For this review, take the finished solid that the model builds, in its own axes (mm). A direction names the side the tool comes from. Give positions to 0.01 mm unless a question says otherwise; leave off trailing zeros. Order: outer loops, then holes, each group sorted by start corner. A loop starts at its lowest first (then second) coordinate and runs counter-clockwise, first axis right, second up. Notation, with made-up numbers: (31, 71.25) - (47, 71.25) arc R26 cw to (47, 101.25) - close; hole circle Ø1 at (-18.75, -28). An arc over 180 degrees is marked (long way). Answer as a JSON object with one key per item and string values. Group by question number.
from build123d import *

# Parameters (mm, degrees)
F0_R     = 1.5
F0_R_2   = 4.5
F1_DEPTH = 2


with BuildPart() as f1:
    # F0 (on Top) → F1 (new body)
    with BuildSketch(Plane.XY):
        with BuildLine():
            ThreePointArc((-8.332531, 2.986763), (-11.332531, -0.013237), (-8.332531, -3.013237))
            Line((-8.332531, -3.013237), (-7.332531, -3.013237))
            ThreePointArc((-7.332531, -3.013237), (-4.504103, -4.184809), (-3.332531, -7.013237))
            Line((-3.332531, -7.013237), (-3.332531, -8.013237))
            ThreePointArc((-3.332531, -8.013237), (-0.332531, -11.013237), (2.667469, -8.013237))
            Line((2.667469, -8.013237), (2.667469, -7.013237))
            ThreePointArc((2.667469, -7.013237), (3.839042, -4.184809), (6.667469, -3.013237))
            Line((6.667469, -3.013237), (7.667469, -3.013237))
            ThreePointArc((7.667469, -3.013237), (10.667469, -0.013237), (7.667469, 2.986763))
            Line((7.667469, 2.986763), (6.667469, 2.986763))
            ThreePointArc((6.667469, 2.986763), (3.839042, 4.158336), (2.667469, 6.986763))
            Line((2.667469, 6.986763), (2.667469, 7.986763))
            ThreePointArc((2.667469, 7.986763), (-0.332531, 10.986763), (-3.332531, 7.986763))
            Line((-3.332531, 7.986763), (-3.332531, 6.986763))
            ThreePointArc((-3.332531, 6.986763), (-4.504103, 4.158336), (-7.332531, 2.986763))
            Line((-7.332531, 2.986763), (-8.332531, 2.986763))
        make_face()
        with Locations((-0.332531, -8.013237)):
            Circle(F0_R, mode=Mode.SUBTRACT)
        with Locations((-8.332531, -0.013237)):
            Circle(F0_R, mode=Mode.SUBTRACT)
        with Locations((-0.332531, -0.013237)):
            Circle(F0_R_2, mode=Mode.SUBTRACT)
        with Locations((7.667469, -0.013237)):
            Circle(F0_R, mode=Mode.SUBTRACT)
        with Locations((-0.332531, 7.986763)):
            Circle(F0_R, mode=Mode.SUBTRACT)
    extrude(amount=F1_DEPTH)


solid = f1.part
1) For line 1 (Y direction, x = -1, z = 1.4); line 2 (X direction, y = 0.5, z = 0.8); line 3 (X direction, y = 1, z = 1.85), list the stretches that pass through material, from the lowest coordinate up.
2) Mouldability with a two-part tool opening along Y and no side actions: class faces 1 (the face through (-4.54, -4.15, 0.99)), 2 (the face through (-9.83, 0.05, 0.99)), 3 (the face through (7, 2.987, 1)), 4 (the face through (2.1, 4.1, 0)) as released by +Y, released by -Y, zero draft, split by the parting line, or undercut.
3) For pin 1 (2.5 mm diameter, centred on x = -8.33, y = -0.01, fed in from -Z); pin 2 (1.1 mm diameter, centred on x = -8, z = 1, fed in from +Y); pin 3 (0.8 mm diameter, centred on y = 7.5, z = 1.5, fed in from +X); pin 4 (1.1 mm diameter, centred on y = 7.5, z = 1, fed in from -X), all flat-tipped, find the tip position at first contact; note any pin that passes through.
4) Consider section C-C (z = 1.2). Give the boundary of the cut face in (x, y), plus the area to 3 significant figures.
5) For faces 5 (the face through (7, -3.013, 1)), 6 (the face through (-3.333, 7.5, 1)), 7 (the face through (-8, -3.013, 1)), list the 3-axis set-ups (+Z, -Z, +X, -X, +Y, -Y) from which the entire face can be reached by the end or side of a thin tool; tool diameter is ignored.
6) Consider section D-D (y = -4.25). Give the boundary of the cut face in (x, z).
7) Consider section B-B (y = 0.75). Give the boundary of the cut face in (x, z), plus the area to 3 significant figures.
8) Consider section A-A (x = -3.75). Give the boundary of the cut face in (y, z).
Result set:
{
 "1": {"line 1": "y = -10.94 to -9.36, -6.67 to -4.46, 4.44 to 6.64, 9.33 to 10.91", "line 2": "x = -11.29 to -9.74, -6.92 to -4.8, 4.14 to 6.26, 9.08 to 10.62", "line 3": "x = -11.16 to -9.44, -7.23 to -4.72, 4.05 to 6.56, 8.77 to 10.49"},
 "2": {"face 1": "released by -Y", "face 2": "undercut", "face 3": "released by +Y", "face 4": "zero draft"},
 "3": {"pin 1": "passes through", "pin 2": "stops at y = 2.99", "pin 3": "stops at x = 2.67", "pin 4": "stops at x = -3.33"},
 "4": {"outline": "(-8.33, -3.01) - (-7.33, -3.01) arc R4 cw to (-3.33, -7.01) - (-3.33, -8.01) arc R3 ccw to (2.67, -8.01) - (2.67, -7.01) arc R4 cw to (6.67, -3.01) - (7.67, -3.01) arc R3 ccw to (7.67, 2.99) - (6.67, 2.99) arc R4 cw to (2.67, 6.99) - (2.67, 7.99) arc R3 ccw to (-3.33, 7.99) - (-3.33, 6.99) arc R4 cw to (-7.33, 2.99) - (-8.33, 2.99) arc R3 ccw to start; hole circle Ø3 at (-8.33, -0.01); hole circle Ø9 at (-0.33, -0.01); hole circle Ø3 at (-0.33, -8.01); hole circle Ø3 at (-0.33, 7.99); hole circle Ø3 at (7.67, -0.01)", "area": "134 mm2"},
 "5": {"face 5": "+Z, -Z, +X, -Y", "face 6": "+Z, -Z, -X, +Y", "face 7": "+Z, -Z, -X, -Y"},
 "6": {"outline": "(-4.44, 0) - (-1.85, 0) - (-1.85, 2) - (-4.44, 2) - close; (1.18, 0) - (3.78, 0) - (3.78, 2) - (1.18, 2) - close"},
 "7": {"outline": "(-11.23, 0) - (-9.62, 0) - (-9.62, 2) - (-11.23, 2) - close; (-7.04, 0) - (-4.77, 0) - (-4.77, 2) - (-7.04, 2) - close; (4.1, 0) - (6.38, 0) - (6.38, 2) - (4.1, 2) - close; (8.96, 0) - (10.57, 0) - (10.57, 2) - (8.96, 2) - close", "area": "15.5 mm2"},
 "8": {"outline": "(-5.23, 0) - (-2.94, 0) - (-2.94, 2) - (-5.23, 2) - close; (2.91, 0) - (5.21, 0) - (5.21, 2) - (2.91, 2) - close"}
}
